Geometry: final body of the model. Coordinates: model frame, mm. A direction names the side the tool comes from. Give positions to 0.01 mm unless a question says otherwise; leave off trailing zeros. Order: outer loops, then holes, each group sorted by start corner. A loop starts at its lowest first (then second) coordinate and runs counter-clockwise, first axis right, second up. Notation, with made-up numbers: (-29, -17.5) - (12, -17.5) arc R12 cw to (12, -9.5) - close; hole circle Ø2 at (43, 67.25). An arc over 180 degrees is marked (long way). Put each result on its own line as item: value. Start each with the question number.
1. Section C-C on x = -86.5. Return the cut outline in (y, z), plus the area to 3 significant figures.
2. Section A-A on z = 20. Return the cut outline in (x, y), plus the area to 3 significant figures.
3. Section B-B on y = 8.5. Return the cut outline in (x, z), plus the area to 3 significant figures.
4. Ray query, line 1 along X through (y, z) = (-11, -23); line 2 along Z through (x, y) = (-63.5, -27); line 3 along Y through (x, z) = (-98.5, -1.5). Return the intervals inside material, ascending. Write a range as from..to.
5. Set-up query: faces 5 (the flat face through (78.471, 0, -21)), 6 (the flat face through (-1, 1, 11.866)), 7 (the flat face through (104, -28.016, -2)). Return all of +Z, -Z, +X, -X, +Y, -Y with unobstructed straight access to the full face (end or side cutting, diameter ignored); none if empty.
6. First-contact query: P1, Ø9.5, axis at y = -36.5, z = 5, coming from the +X side; P2, Ø15.5, axis at x = 116, z = -12, coming from the +Y side; P3, Ø5.5, axis at y = -35, z = 4, coming from the -X side. Flat tips, straight axial feed; report the tip coordinate or a pass-through.
7. Mould query, pull axis X, two halves, no side actions, for faces 1 (the flat face through (-1, 1, 0)), 2 (the flat face through (104, 28.016, -2)), 3 (the flat face through (-78.471, 0, -25)), 4 (the flat face through (-134.405, 0, -7)). Classes: pulls with the +X half, pulls with the -X half, needs draft (parallel to the pull), parting line crosses it, or undercut.
8. Section D-D on x = 17.5. Return the cut outline in (y, z), plus the area to 3 significant figures.
from build123d import *

# Parameters (mm, degrees)
F0_W          = 156.942024
F0_H          = 80.822982
F1_DEPTH      = 11.86577
F2_W          = 55.933565
F2_H          = 58.87492
F4_DEPTH      = 24.27763
F4_DEPTH_BACK = 62.99935
F3_W          = 52.396328
F3_H          = 56.031708
F5_DEPTH      = 25.4
F5_DEPTH_BACK = 54.0204


with BuildPart() as f1:
    # F0 (on Top) → F1 (new body)
    with BuildSketch(Plane.XY):
        Rectangle(F0_W, F0_H)
    extrude(amount=F1_DEPTH)

    # F2 (on face) → F4 (join, two sides)
    with BuildSketch(Plane.XY.offset(11.86577)) as f4_sk:
        with Locations((-106.437794, 0)):
            Rectangle(F2_W, F2_H)
    extrude(amount=F4_DEPTH)
    extrude(f4_sk.sketch, amount=-F4_DEPTH_BACK)

    # F3 (on face) → F5 (join, two sides)
    with BuildSketch(Plane.XY.offset(11.86577)) as f5_sk:
        with Locations((104.669176, 0)):
            Rectangle(F3_W, F3_H)
    extrude(amount=F5_DEPTH)
    extrude(f5_sk.sketch, amount=-F5_DEPTH_BACK)


solid = f1.part
Resolved:
1. outline: (-29.44, -51.13) - (29.44, -51.13) - (29.44, 36.14) - (-29.44, 36.14) - close
1. area: 5,140 mm^2
2. outline: (-134.4, -29.44) - (-78.47, -29.44) - (-78.47, 29.44) - (-134.4, 29.44) - close; (78.47, -28.02) - (130.87, -28.02) - (130.87, 28.02) - (78.47, 28.02) - close
2. area: 6,230 mm^2
3. outline: (-134.4, -51.13) - (-78.47, -51.13) - (-78.47, 0) - (78.47, 0) - (78.47, -42.15) - (130.87, -42.15) - (130.87, 37.27) - (78.47, 37.27) - (78.47, 11.87) - (-78.47, 11.87) - (-78.47, 36.14) - (-134.4, 36.14) - close
3. area: 10,900 mm^2
4. line 1: -134.4..-78.47, 78.47..130.87
4. line 2: 0..11.87
4. line 3: -29.44..29.44
5. face 5: -Z, +Y, -Y
5. face 6: +Z, +Y, -Y
5. face 7: +Z, -Z, +X, -Y
6. P1: x = 78.47
6. P2: y = 28.02
6. P3: x = -78.47
7. face 1: undercut
7. face 2: needs draft
7. face 3: undercut
7. face 4: pulls with the -X half
8. outline: (-40.41, 0) - (40.41, 0) - (40.41, 11.87) - (-40.41, 11.87) - close
8. area: 959 mm^2
